The listing builds one solid part. Answer for the finished solid, in the listing's coordinates (mm). A direction names the side the tool comes from. Coordinates: 2 decimals unless noted, no trailing zeros. Write each loop counter-clockwise with the first axis right and the second up, starting at its lowest first coordinate (ties: lowest second). Pieces come first, ordered by that corner, then holes.
from build123d import *

# Parameters (mm, degrees)
PAD_DEPTH           = 17.5
SKETCH001_R         = 1.6
POCKET_DEPTH        = 30.001
POCKET_DEPTH_BACK   = 30.001
SKETCH009_R         = 2.1
POCKET002_DEPTH     = 10
POCKET006_DEPTH     = 1.5
SKETCH014_R         = 1.8
HOLE_DEPTH          = 10
HOLE001_D           = 3.2
HOLE001_DEPTH       = 9
HOLE001_CBORE_D     = 3.3
HOLE001_CBORE_DEPTH = 3.5
HOLE001_TIPS_R      = 1.6
HOLE002_D           = 3.2
HOLE002_DEPTH       = 9
HOLE002_CBORE_D     = 3.3
HOLE002_CBORE_DEPTH = 3.5
HOLE002_TIPS_R      = 1.6
SKETCH018_W         = 1
SKETCH018_H         = 7.240904
SKETCH018_H_2       = 8.067387
POCKET009_DEPTH     = 10
SKETCH019_W         = 1
SKETCH019_H         = 13.038261
SKETCH019_H_2       = 12.983065
POCKET010_DEPTH     = 10
FILLET_R            = 1


with BuildPart() as part:
    # Sketch → Pad (new body, symmetric)
    with BuildSketch(Plane.XZ):
        Polygon((-30, 20), (-30, 0), (30, 0), (30, 20), (22, 20), (22, 8), (-22, 8), (-22, 20), align=None)
    extrude(amount=PAD_DEPTH, both=True)

    # Sketch001 → Pocket (cut, two sides)
    with BuildSketch(Plane.YZ) as pocket_sk:
        with Locations((-13.5, 14)):
            Circle(SKETCH001_R)
        with Locations((13.5, 14)):
            Circle(SKETCH001_R)
    extrude(amount=-POCKET_DEPTH, mode=Mode.SUBTRACT)
    extrude(pocket_sk.sketch, amount=POCKET_DEPTH_BACK, mode=Mode.SUBTRACT)

    # Sketch009 (on DatumPlane) → Pocket002 (cut)
    with BuildSketch(Plane.YZ.offset(30)):
        with Locations((-4.5, 14)):
            Circle(SKETCH009_R)
        with Locations((4.5, 14)):
            Circle(SKETCH009_R)
    extrude(amount=-POCKET002_DEPTH, mode=Mode.SUBTRACT)

    # Sketch013 (on DatumPlane) → Pocket006 (cut)
    with BuildSketch(Plane.YZ.offset(30)):
        with BuildLine():
            ThreePointArc((-0.929111, 16.156676), (-0.929111, 17.570889), (-2.343324, 17.570889))
            Line((-2.343324, 17.570889), (-8.070889, 11.843324))
            ThreePointArc((-8.070889, 11.843324), (-8.070889, 10.429111), (-6.656676, 10.429111))
            Line((-6.656676, 10.429111), (-0.929111, 16.156676))
        make_face()
        with BuildLine():
            ThreePointArc((2.343324, 17.570889), (0.929111, 17.570889), (0.929111, 16.156676))
            Line((0.929111, 16.156676), (6.656676, 10.429111))
            ThreePointArc((6.656676, 10.429111), (8.070889, 10.429111), (8.070889, 11.843324))
            Line((8.070889, 11.843324), (2.343324, 17.570889))
        make_face()
    extrude(amount=-POCKET006_DEPTH, mode=Mode.SUBTRACT)

    # Sketch014 (on DatumPlane) → Hole (cut)
    with BuildSketch(Plane.YZ.offset(-30)):
        with Locations((0, 14)):
            Circle(SKETCH014_R)
    extrude(amount=HOLE_DEPTH, mode=Mode.SUBTRACT)

    # Hole001
    with Locations(Plane.XZ.offset(17.5)):
        with Locations((26, 17.441701), (-26, 17.441701)):
            CounterBoreHole(HOLE001_D / 2, HOLE001_CBORE_D / 2, HOLE001_CBORE_DEPTH, depth=HOLE001_DEPTH)

    # Hole001 tips → Hole001 tip 1 section 0
    with BuildSketch(Plane.XZ.offset(8.5), mode=Mode.PRIVATE) as hole001_tip_1_s0:
        with Locations((26, 17.441701)):
            Circle(HOLE001_TIPS_R)
    loft([hole001_tip_1_s0.sketch, Vertex(26, -7.538623, 17.441701)], mode=Mode.SUBTRACT)

    # Hole001 tips → Hole001 tip 2 section 0
    with BuildSketch(Plane.XZ.offset(8.5), mode=Mode.PRIVATE) as hole001_tip_2_s0:
        with Locations((-26, 17.441701)):
            Circle(HOLE001_TIPS_R)
    loft([hole001_tip_2_s0.sketch, Vertex(-26, -7.538623, 17.441701)], mode=Mode.SUBTRACT)

    # Hole002
    with Locations(Plane(origin=(0, 17.5, 0), x_dir=(-1, 0, 0), z_dir=(0, 1, 0))):
        with Locations((-26, 17.441701), (26, 17.441701)):
            CounterBoreHole(HOLE002_D / 2, HOLE002_CBORE_D / 2, HOLE002_CBORE_DEPTH, depth=HOLE002_DEPTH)

    # Hole002 tips → Hole002 tip 1 section 0
    with BuildSketch(Plane(origin=(0, 8.5, 0), x_dir=(-1, 0, 0), z_dir=(0, 1, 0)), mode=Mode.PRIVATE) as hole002_tip_1_s0:
        with Locations((-26, 17.441701)):
            Circle(HOLE002_TIPS_R)
    loft([hole002_tip_1_s0.sketch, Vertex(26, 7.538623, 17.441701)], mode=Mode.SUBTRACT)

    # Hole002 tips → Hole002 tip 2 section 0
    with BuildSketch(Plane(origin=(0, 8.5, 0), x_dir=(-1, 0, 0), z_dir=(0, 1, 0)), mode=Mode.PRIVATE) as hole002_tip_2_s0:
        with Locations((26, 17.441701)):
            Circle(HOLE002_TIPS_R)
    loft([hole002_tip_2_s0.sketch, Vertex(-26, 7.538623, 17.441701)], mode=Mode.SUBTRACT)

    # Sketch018 (on DatumPlane) → Pocket009 (cut)
    with BuildSketch(Plane.YZ.offset(-30)):
        with Locations((-13.5, 17.620452)):
            Rectangle(SKETCH018_W, SKETCH018_H)
        with Locations((13.5, 18.033693)):
            Rectangle(SKETCH018_W, SKETCH018_H_2)
    extrude(amount=POCKET009_DEPTH, mode=Mode.SUBTRACT)

    # Sketch019 (on DatumPlane) → Pocket010 (cut)
    with BuildSketch(Plane.YZ.offset(30)):
        with Locations((-13.5, 20.51913)):
            Rectangle(SKETCH019_W, SKETCH019_H)
        with Locations((13.5, 20.491532)):
            Rectangle(SKETCH019_W, SKETCH019_H_2)
    extrude(amount=-POCKET010_DEPTH, mode=Mode.SUBTRACT)

    # Fillet
    fillet_edges = [part.edges().sort_by_distance(p)[0] for p in [
        (0, 17.5, 0),
        (-30, 0, 0),
        (0, -17.5, 0),
        (30, 0, 0),
    ]]
    fillet(fillet_edges, radius=FILLET_R)


solid = part.part
Q1. Find the intervals of material crossed by probe 1 along Y at (x, z) = (-22.5, 16); probe 2 along X at (y, z) = (0.5, 11); probe 3 along Z at (x, y) = (-26, 16.05), in increasing order.
Answers below:
probe 1: y = -17.5 to -14, -13 to 13, 14 to 17.5
probe 2: x = -30 to -22, 22 to 30
probe 3: z = 0 to 15.79, 19.09 to 20
Q2. The part is cut by section A-A, the plane y = 4.5. Write down the section's boundary in (x, z), then the cut area to 3 significant figures.
Answers below:
outline: (-30, 1) arc R1 ccw to (-29, 0) - (29, 0) arc R1 ccw to (30, 1) - (30, 11.9) - (22, 11.9) - (22, 8) - (-22, 8) - (-22, 20) - (-30, 20) - close; (22, 16.1) - (30, 16.1) - (30, 20) - (22, 20) - close
area: 638 mm2
Q3. The part is cut by section D-D, the plane y = 0. Write down the section's boundary in (x, z).
Answers below:
outline: (-30, 1) arc R1 ccw to (-29, 0) - (29, 0) arc R1 ccw to (30, 1) - (30, 20) - (22, 20) - (22, 8) - (-22, 8) - (-22, 12.2) - (-30, 12.2) - close; (-30, 15.8) - (-22, 15.8) - (-22, 20) - (-30, 20) - close
Q4. The part is cut by section C-C, the plane x = 15. Write down the section's boundary in (y, z), then the cut area to 3 significant figures.
Answers below:
outline: (-17.5, 1) arc R1 ccw to (-16.5, 0) - (16.5, 0) arc R1 ccw to (17.5, 1) - (17.5, 8) - (-17.5, 8) - close
area: 280 mm2
Q5. The part is cut by section B-B, the plane z = 11.25. Write down the section's boundary in (x, y), then the cut area to 3 significant figures.
Answers below:
outline: (-30, -17.5) - (-22, -17.5) - (-22, 17.5) - (-30, 17.5) - close; (22, -17.5) - (30, -17.5) - (30, -8.36) - (28.5, -8.36) - (28.5, -5.84) - (30, -5.84) - (30, 5.84) - (28.5, 5.84) - (28.5, 8.36) - (30, 8.36) - (30, 17.5) - (22, 17.5) - close
area: 552 mm2
Q6. Which of the six approach directions +Z, -Z, +X, -X, +Y, -Y give full straight-line access (tool end or side, diameter ignored) to faces 1 (the face through (-26.056, -0.234, 15.785)), 2 (the face through (26.1, -13, 19.2)), 3 (the face through (-26.208, 10.718, 19.028)), 4 (the face through (26.056, -6.166, 12.722))?
Answers below:
face 1: -X
face 2: +Z, +X, -X
face 3: +Y
face 4: +X
Q7. Determine the mould class of faces 5 (the face through (-24.784, 15.774, 18.557)), 6 (the face through (-26.2, -7.69, 17.29)), 7 (the face through (29.26, 1.697, 15.389)), 8 (the face through (-26.1, 13, 19.2)) for opening direction Y: released by +Y, released by -Y, zero draft, split by the parting line, or undercut.
Answers below:
face 5: zero draft
face 6: released by -Y
face 7: undercut
face 8: undercut
Q8. Given pin 1 (10.5 mm diameter, centred on x = 6.5, y = 7, fed in from +Z); pin 2 (2.5 mm diameter, centred on x = 26, z = 17.44, fed in from -Y), each flat-ended and moving along its own axis, determine where each tip first touches the part or whether it passes through.
Answers below:
pin 1: stops at z = 8
pin 2: stops at y = -8.29
